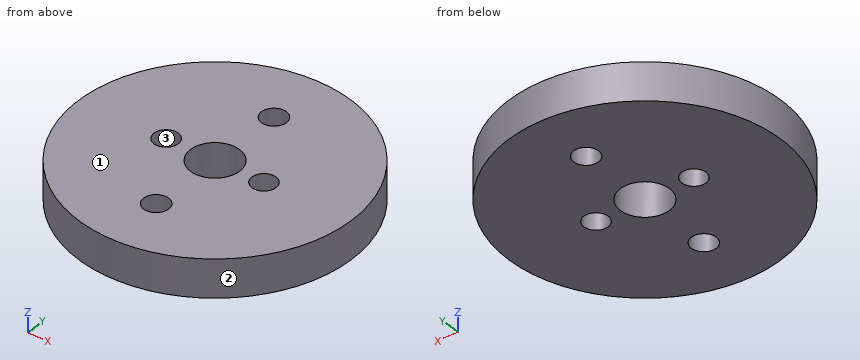
from build123d import *

# Parameters (mm, degrees)
SKETCH_1_R          = 18
SKETCH_1_R_2        = 3.25
SKETCH_1_R_3        = 1.6
EXTRUDE_1_DEPTH     = 5
SKETCH_2_R          = 1.65
CUT_EXTRUDE_1_DEPTH = 26.942243542


with BuildPart() as part:
    # ｽｹｯﾁ1 → ﾎﾞｽ - 押し出し1 (new body)
    with BuildSketch(Plane.XY):
        Circle(SKETCH_1_R)
        Circle(SKETCH_1_R_2, mode=Mode.SUBTRACT)
        with Locations((6.5, 0)):
            Circle(SKETCH_1_R_3, mode=Mode.SUBTRACT)
        with Locations(Location((-6.5, 0, 0), (0, 0, 180))):
            Circle(SKETCH_1_R_3, mode=Mode.SUBTRACT)
    extrude(amount=EXTRUDE_1_DEPTH)

    # ｽｹｯﾁ2 → ｶｯﾄ - 押し出し1 (cut, through all)
    with BuildSketch(Plane.XY.offset(5)):
        with Locations((0, 10)):
            Circle(SKETCH_2_R)
        with Locations(Location((0, -10, 0), (0, 0, 180))):
            Circle(SKETCH_2_R)
    extrude(amount=-CUT_EXTRUDE_1_DEPTH, mode=Mode.SUBTRACT)


solid = part.part
Verification items for the finished model (mm, model axes). Face numbers are marked on the shaded views. Round coordinates to 2 decimals unless told otherwise and drop trailing zeros. Loops run counter-clockwise (first coordinate to the right, second up) from the corner with the lowest first, then second, coordinate; pieces in that order, holes last. Notation, with made-up numbers: (73, 76) - (121, 76) arc R7 ccw to (121, 82) - close; hole circle Ø1 at (58, -13). An arc over 180 degrees is marked (long way). Use a Markdown table: item, result. Add a question column.
1. Gauge pin test, flat ends, axial feed: pin 1 (12 mm diameter, centred on x = -2, y = -7.5, fed in from -Z); pin 2 (3 mm diameter, centred on y = 13.5, z = 1.5, fed in from +X); pin 3 (2 mm diameter, centred on x = 1, z = 0.5, fed in from +Y); pin 4 (2 mm diameter, centred on x = 0, y = 10, fed in from +Z). Record the tip position at first contact, or that the pin passes through.
2. Section check D-D, the plane z = 4.25. Record the boundary of the cut face in (x, y), plus the area to 4 significant figures.
3. Thickness scan on probe 1 along Y at (x, z) = (0, 1.15); probe 2 along Y at (x, z) = (-6.5, 2.85); probe 3 along Y at (x, z) = (7, 2.75). Record the ranges inside material, lowest first. Write a range as [from, to].
4. Release check for a two-part mould opening along Y. For the marked faces 1, 2 and 3 record: released by +Y, released by -Y, zero draft, split by the parting line, or undercut.
5. Section check B-B, the plane y = -10. Record the boundary of the cut face in (x, z).
6. Section check C-C, the plane x = 7. Record the boundary of the cut face in (y, z).
7. Section check A-A, the plane y = 0. Record the boundary of the cut face in (x, z).
Checks:
| question | item | result |
|---|---|---|
| 1 | pin 1 | stops at z = 0 |
| 1 | pin 2 | stops at x = 13.42 |
| 1 | pin 3 | stops at y = 18 |
| 1 | pin 4 | passes through |
| 2 | outline | circle Ø36 at (0, 0); hole circle Ø3.2 at (-6.5, 0); hole circle Ø6.5 at (0, 0); hole circle Ø3.3 at (0, -10); hole circle Ø3.3 at (0, 10); hole circle Ø3.2 at (6.5, 0) |
| 2 | area | 951.5 mm^2 |
| 3 | probe 1 | y = [-18, -11.65], [-8.35, -3.25], [3.25, 8.35], [11.65, 18] |
| 3 | probe 2 | y = [-16.79, -1.6], [1.6, 16.79] |
| 3 | probe 3 | y = [-16.58, -1.52], [1.52, 16.58] |
| 4 | face 1 | zero draft |
| 4 | face 2 | split by the parting line |
| 4 | face 3 | undercut |
| 5 | outline | (-14.97, 0) - (-1.65, 0) - (-1.65, 5) - (-14.97, 5) - close; (1.65, 0) - (14.97, 0) - (14.97, 5) - (1.65, 5) - close |
| 6 | outline | (-16.58, 0) - (-1.52, 0) - (-1.52, 5) - (-16.58, 5) - close; (1.52, 0) - (16.58, 0) - (16.58, 5) - (1.52, 5) - close |
| 7 | outline | (-18, 0) - (-8.1, 0) - (-8.1, 5) - (-18, 5) - close; (-4.9, 0) - (-3.25, 0) - (-3.25, 5) - (-4.9, 5) - close; (3.25, 0) - (4.9, 0) - (4.9, 5) - (3.25, 5) - close; (8.1, 0) - (18, 0) - (18, 5) - (8.1, 5) - close |
